from build123d import *

# Parameters (mm, degrees)
BOSS_EXTRUDE1_DEPTH      = 13.6
FILLET1_R                = 2.54
BOSS_EXTRUDE2_DEPTH      = 0.5
BOSS_EXTRUDE2_DEPTH_BACK = 34.8
SKETCH3_R                = 5.5
CUT_EXTRUDE2_DEPTH       = 51.336393456


with BuildPart() as part:
    # Sketch1 → Boss-Extrude1 (new body)
    with BuildSketch(Plane(origin=(0, 0, 0), x_dir=(1, 0, 0), z_dir=(0, 1, 0))):
        with BuildLine():
            Line((-23.519969056, 17.15), (23.519969056, 17.15))
            ThreePointArc((23.519969056, 17.15), (28.255759205, 15.304831876), (30.494883917, 10.742083333))
            ThreePointArc((30.494883917, 10.742083333), (30.95, 0), (30.494883917, -10.742083333))
            ThreePointArc((30.494883917, -10.742083333), (28.255759205, -15.304831876), (23.519969056, -17.15))
            Line((23.519969056, -17.15), (-23.519969056, -17.15))
            ThreePointArc((-23.519969056, -17.15), (-28.255759205, -15.304831876), (-30.494883917, -10.742083333))
            ThreePointArc((-30.494883917, -10.742083333), (-30.95, 0), (-30.494883917, 10.742083333))
            ThreePointArc((-30.494883917, 10.742083333), (-28.255759205, 15.304831876), (-23.519969056, 17.15))
        make_face()
    extrude(amount=BOSS_EXTRUDE1_DEPTH)

    # Fillet1
    fillet1_edges = [part.edges().sort_by_distance(p)[0] for p in [
        (-30.95, 0, 0),
        (-28.255759205, 0, -15.304831876),
        (0, 0, -17.15),
        (28.255759205, 0, -15.304831876),
        (30.95, 0, 0),
        (28.255759205, 0, 15.304831876),
        (0, 0, 17.15),
        (-28.255759205, 0, 15.304831876),
    ]]
    fillet(fillet1_edges, radius=FILLET1_R)

    # Sketch3 → Boss-Extrude2 (add, two sides: drawn at the far end of the back side and taken through both)
    with BuildSketch(Plane.XY.offset(17.15).offset(-BOSS_EXTRUDE2_DEPTH_BACK)):
        with Locations((-17.438993952, 13.6)):
            Circle(SKETCH3_R)
    extrude(amount=BOSS_EXTRUDE2_DEPTH + BOSS_EXTRUDE2_DEPTH_BACK)

    # Sketch5 → Cut-Extrude2 (cut, through all)
    with BuildSketch(Plane.XY.offset(17.15)):
        Polygon((-22.938993952, 13.6), (-30.95, 11.453457399), (-30.95, 13.6), align=None)
    extrude(amount=-CUT_EXTRUDE2_DEPTH, mode=Mode.SUBTRACT)


solid = part.part
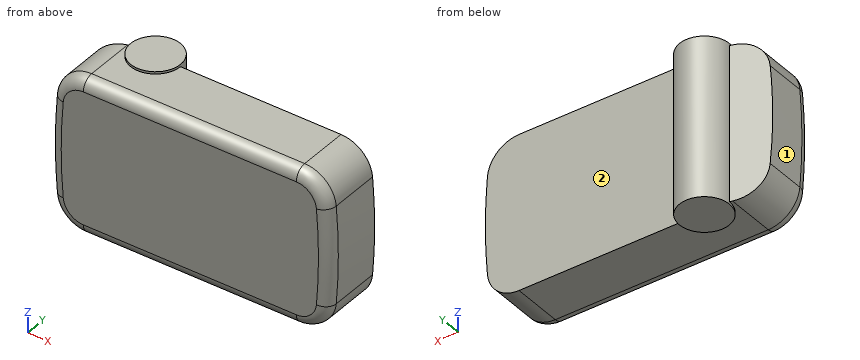
Could you check a few things on this model? Use its own coordinates, in mm. Face numbers are marked on the shaded views. A direction names the side the tool comes from. Give positions to 0.01 mm unless a question says otherwise; leave off trailing zeros. Order: outer loops, then holes, each group sorted by start corner. A loop starts at its lowest first (then second) coordinate and runs counter-clockwise, first axis right, second up.
Item 1: I need wall thicknesses on line 1 (Z direction, x = -20.5, y = 4.25); line 2 (Y direction, x = -3, z = 7); line 3 (X direction, y = 3.5, z = 1). Which ranges of each line are inside material? Lowest first, please.
Item 2: If we section it at B-B, the plane x = 2: Write out the boundary of the cut face in (y, z), plus the area to 3 significant figures.
Item 3: If we section it at A-A, the plane x = -21.5: Write out the boundary of the cut face in (y, z).
Item 4: I'm going to push flat-ended pins straight in: pin 1 (1.5 mm diameter, centred on x = 10, z = -7, fed in from +Y); pin 2 (1 mm diameter, centred on x = 20.5, y = 12.5, fed in from +Z); pin 3 (1.5 mm diameter, centred on x = -2.5, y = 14.5, fed in from -Z); pin 4 (5 mm diameter, centred on y = 8, z = 3.5, fed in from -X). Where does each tip first touch, or does it pass through?
Item 5: For the marked faces 1 and 2, which set-ups out of +Z, -Z, +X, -X, +Y, -Y let a thin tool reach every point of the face, with its end or its side?
Item 6: If we section it at C-C, the plane y = 17.25: Write out the boundary of the cut face in (x, z), plus the area to 3 significant figures.
Values:
1. line 1: z = -17.15 to 17.15
1. line 2: y = 0 to 13.6
1. line 3: x = -30.95 to 30.95
2. outline: (0, -14.61) arc R2.54 ccw to (2.54, -17.15) - (13.6, -17.15) - (13.6, 17.15) - (2.54, 17.15) arc R2.54 ccw to (0, 14.61) - close
2. area: 464 mm2
3. outline: (0, -14.61) arc R2.54 ccw to (2.54, -17.15) - (9.89, -17.15) - (9.89, -17.65) - (17.31, -17.65) - (17.31, 17.65) - (9.89, 17.65) - (9.89, 17.15) - (2.54, 17.15) arc R2.54 ccw to (0, 14.61) - close
4. pin 1: stops at y = 13.6
4. pin 2: stops at z = 17.15
4. pin 3: passes through
4. pin 4: stops at x = -30.95
5. face 1: -X, +Y, -Y
5. face 2: +Z, -Z, +X, +Y
6. outline: (-21.55, -17.65) - (-13.32, -17.65) - (-13.32, 17.65) - (-21.55, 17.65) - close
6. area: 290 mm2
